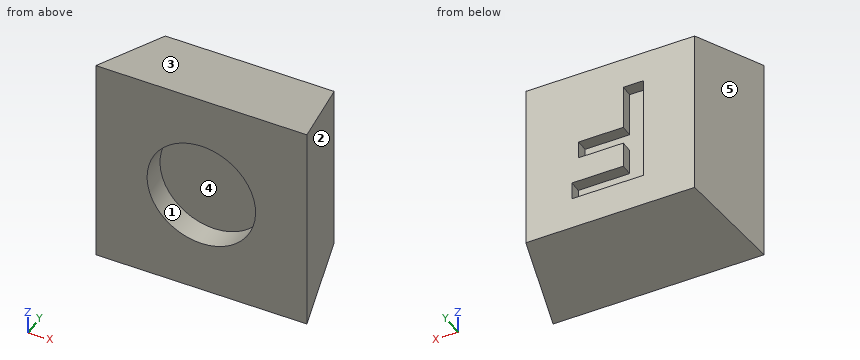
from build123d import *

# Parameters (mm, degrees)
SKETCH1_W           = 7
SKETCH1_H           = 7
BOSS_EXTRUDE1_DEPTH = 3
CUT_EXTRUDE1_DEPTH  = 7
CUT_EXTRUDE2_DEPTH  = 11
SKETCH4_R           = 1.8
CUT_EXTRUDE3_DEPTH  = 0.8
CUT_EXTRUDE4_DEPTH  = 0.4


with BuildPart() as part:
    # Sketch1 → Boss-Extrude1 (new body)
    with BuildSketch(Plane(origin=(0, 0, 0), x_dir=(1, 0, 0), z_dir=(0, 1, 0))):
        with Locations((3.5, 3.5)):
            Rectangle(SKETCH1_W, SKETCH1_H)
    extrude(amount=BOSS_EXTRUDE1_DEPTH)

    # Sketch2 → Cut-Extrude1 (cut)
    with BuildSketch(Plane.XY):
        Polygon((0, 0), (0.7, 3), (0, 3), align=None)
        Polygon((7, 0), (6.3, 3), (7, 3), align=None)
    extrude(amount=-CUT_EXTRUDE1_DEPTH, mode=Mode.SUBTRACT)

    # Sketch3 → Cut-Extrude2 (cut)
    with BuildSketch(Plane(origin=(0, 0, 0), x_dir=(0, 0, -1), z_dir=(1, 0, 0))):
        Polygon((0, 0), (0.7, 3), (0, 3), align=None)
        Polygon((7, 3), (6.3, 3), (7, 0), align=None)
    extrude(amount=CUT_EXTRUDE2_DEPTH, mode=Mode.SUBTRACT)

    # Sketch4 → Cut-Extrude3 (cut)
    with BuildSketch(Plane.XZ):
        with Locations(Location((3.5, -3.5, 0), (0, 0, 270))):
            Circle(SKETCH4_R)
    extrude(amount=-CUT_EXTRUDE3_DEPTH, mode=Mode.SUBTRACT)

    # Sketch5 → Cut-Extrude4 (cut)
    with BuildSketch(Plane(origin=(0, 3, 0), x_dir=(1, 0, 0), z_dir=(0, 1, 0))):
        Polygon((2.394882383, 1.732294481), (2.394882383, 5.232294481), (4.773087512, 5.232294481), (4.773087512, 4.648961148), (3.067959306, 4.648961148), (3.067959306, 3.796397045), (4.548728537, 3.796397045), (4.548728537, 3.213063712), (3.067959306, 3.213063712), (3.067959306, 1.732294481), align=None)
    extrude(amount=-CUT_EXTRUDE4_DEPTH, mode=Mode.SUBTRACT)


solid = part.part
Part model, mm, in its own coordinate system. Face numbers are marked on the shaded views. A direction names the side the tool comes from. Round coordinates to 2 decimals unless told otherwise and drop trailing zeros. Write each loop counter-clockwise with the first axis right and the second up, starting at its lowest first coordinate (ties: lowest second). Pieces come first, ordered by that corner, then holes. Notation, with made-up numbers: (26, -9) - (35, -9) arc R10 ccw to (35, -2) - close; hole circle Ø6 at (-31, 72.5). An arc over 180 degrees is marked (long way). Use CSV: the item, a comma, the result in double quotes.
Item 1: Slice it at B-B, the plane z = -3.5. Write the cut outline in (x, y), then the cut area to 3 significant figures.
Results list:
outline,"(0, 0) - (1.7, 0) - (1.7, 0.8) - (5.3, 0.8) - (5.3, 0) - (7, 0) - (6.3, 3) - (4.55, 3) - (4.55, 2.6) - (2.39, 2.6) - (2.39, 3) - (0.7, 3) - close"
area,"15.2 mm²"
Item 2: Flat gauge pins, fed straight in: P1, Ø1.1, axis at x = 3.5, z = -3, coming from the -Y side; P2, Ø3, axis at x = 3.5, z = -3.5, coming from the +Y side; P3, Ø1.5, axis at y = 2, z = -5.5, coming from the -X side; P4, Ø1, axis at x = 2, y = 1, coming from the -Z side. Where does each tip first touch, or does it go through?
Results list:
P1,"stops at y = 0.8"
P2,"stops at y = 3"
P3,"stops at x = 0.29"
P4,"stops at z = -6.88"
Item 3: Slice it at C-C, the plane y = 0.4. Write the cut outline in (x, z).
Results list:
outline,"(0.09, -6.91) - (6.91, -6.91) - (6.91, -0.09) - (0.09, -0.09) - close; hole circle Ø3.6 at (3.5, -3.5)"
Item 4: Slice it at A-A, the plane x = 3.5. Write the cut outline in (y, z).
Results list:
outline,"(0, -7) - (3, -6.3) - (3, -5.23) - (2.6, -5.23) - (2.6, -4.65) - (3, -4.65) - (3, -3.8) - (2.6, -3.8) - (2.6, -3.21) - (3, -3.21) - (3, -0.7) - (0, 0) - (0, -1.7) - (0.8, -1.7) - (0.8, -5.3) - (0, -5.3) - close"
Item 5: Slice it at D-D, the plane y = 2.1. Write the cut outline in (x, z).
Results list:
outline,"(0.49, -6.51) - (6.51, -6.51) - (6.51, -0.49) - (0.49, -0.49) - close"
Item 6: Tool access for the marked faces 1 and 2: list every direction of +Z, -Z, +X, -X, +Y, -Y with a clear straight run to the whole face (end or side of a thin tool).
Results list:
face 1,"-Y"
face 2,"+Z, -Z, +X, +Y"
Item 7: Pull direction X, two halves, no side cores. Call the marked faces 3, 4 and 5: pulls with the +X half, pulls with the -X half, needs draft (parallel to the pull), parting line crosses it, or undercut.
Results list:
face 3,"needs draft"
face 4,"undercut"
face 5,"pulls with the -X half"
Item 8: Wall check: L1, parallel to Z at x = 4.25, y = 2.75; L2, parallel to Y at x = 3, z = -2.75; L3, parallel to X at y = 0.6, z = -3.5. Give the ranges that are in metal, low to high.
Results list:
L1,"z = -6.36 to -5.23, -4.65 to -3.8, -3.21 to -0.64"
L2,"y = 0.8 to 2.6"
L3,"x = 0.14 to 1.7, 5.3 to 6.86"
